Answer from the drawing. Dimensions are ordinates in mm from the lowest x, y and z of the part. Coordinates: 2 decimals unless noted, no trailing zeros. Write each loop counter-clockwise with the first axis right and the second up, starting at its lowest first coordinate (ties: lowest second). Pieces come first, ordered by that corner, then holes.
(1) Straight lines are drawn through the part: line 1 (X direction, y = 1.1, z = 91); line 2 (X direction, y = 1.65, z = 18); line 3 (Z direction, x = 3.5, y = 1.45) (1 decimal). For each, find the intervals that lie inside material, in ascending order.
(2) The part is cut by section C-C on z = 52.5. Determine the outline of the cut face in (x, y).
(3) The part is cut by section D-D on y = 1.65. Give the number of separate pieces and of enclosed holes in the cut face, plus the area to 3 significant figures.
(4) The part is cut by section A-A on z = 25. Determine the outline of the cut face in (x, y).
(5) Given P1, Ø1.5, axis at x = 36, y = 2, coming from the -Z side, flat-ended and moving along its own axis, determine where the tip first touches the part or whether it passes through.
(6) The part is cut by section B-B on x = 9. Determine the outline of the cut face in (y, z).
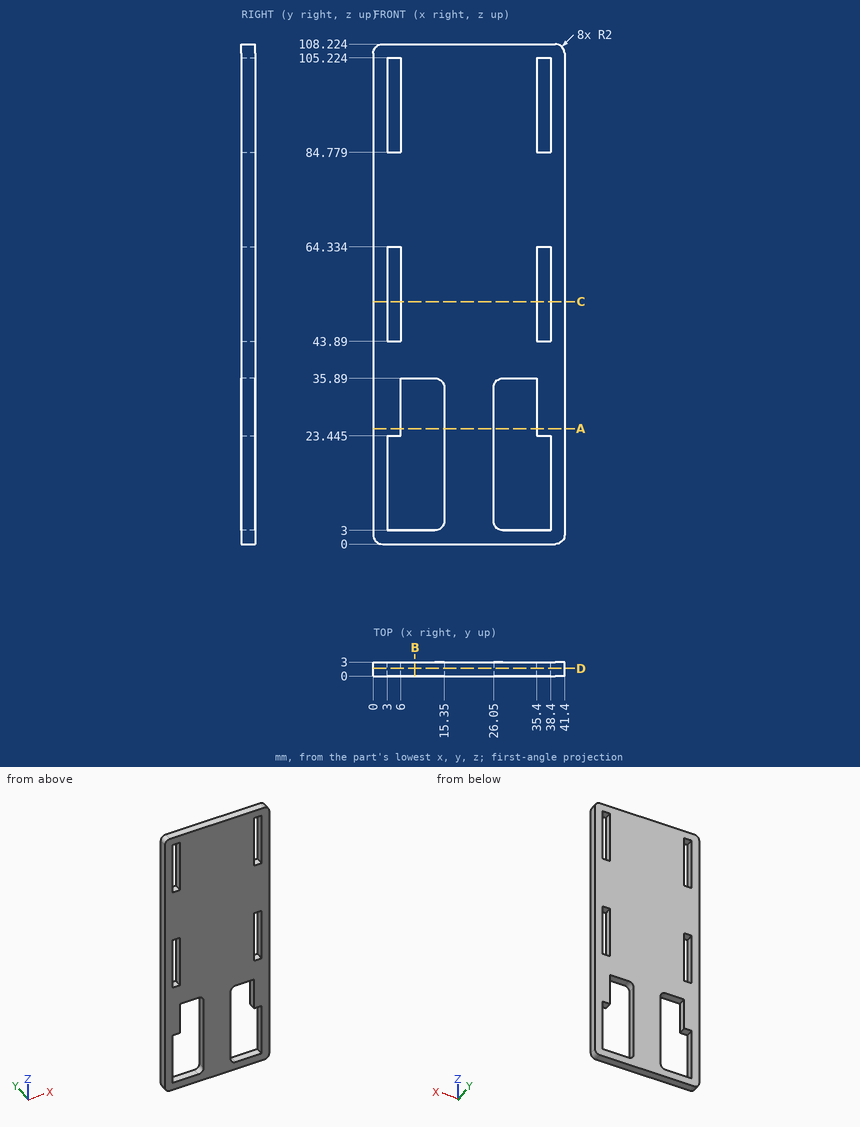
Model answer:
1. line 1: x = 0 to 3, 6 to 35.4, 38.4 to 41.4
1. line 2: x = 0 to 3, 15.35 to 26.05, 38.4 to 41.4
1. line 3: z = 0 to 3, 23.4 to 43.9, 64.3 to 84.8, 105.2 to 108.2
2. outline: (0, 0) - (3, 0) - (3, 3) - (0, 3) - close; (6, 0) - (35.4, 0) - (35.4, 3) - (6, 3) - close; (38.4, 0) - (41.4, 0) - (41.4, 3) - (38.4, 3) - close
3. separate pieces: 1
3. enclosed holes: 6
3. area: 3,500 mm2
4. outline: (0, 0) - (6, 0) - (6, 3) - (0, 3) - close; (15.35, 0) - (26.05, 0) - (26.05, 3) - (15.35, 3) - close; (35.4, 0) - (41.4, 0) - (41.4, 3) - (35.4, 3) - close
5. P1: stops at z = 0
6. outline: (0, 0) - (3, 0) - (3, 3) - (0, 3) - close; (0, 35.89) - (3, 35.89) - (3, 108.22) - (0, 108.22) - close
